Autodesk Inventor part; units mm, degrees
ref_plane "YZ Plane" through (0, 0, 0) normal (1, 0, 0) x (0, 1, 0)
ref_plane "XZ Plane" through (0, 0, 0) normal (0, 1, 0) x (-1, 0, 0)
ref_plane "XY Plane" through (0, 0, 0) normal (0, 0, 1) x (1, 0, 0)
sketch "Sketch1" plane through (0, 0, 0) normal (0, 0, 1) x (1, 0, 0)
  line L0 (-55.88, 39.751) -> (-55.88, -39.751)
  line L1 (-55.88, 39.751) -> (23.622, 39.751) construction
  line L2 (-55.88, -39.751) -> (55.88, -39.751)
  line L3 (55.88, -39.751) -> (55.88, 39.751)
  line L4 (55.88, 39.751) -> (-55.88, 39.751)
  line L5 (0, -55.6514) -> (0, 55.6514)
  line L6 (-78.232, 0) -> (78.232, 0)
  line L7 (-14.351, 39.751) -> (-14.351, 11.049)
  line L8 (-14.351, 11.049) -> (14.351, 11.049)
  line L9 (14.351, 11.049) -> (14.351, 39.751)
  point P0 (0, 0)
  dimension "d0" = 79.502
  dimension "d1" = 90
  dimension "d2" = 111.76
  dimension "d3" = 28.702
  dimension "d4" = 28.702
extrude "Extrusion1" add sketch "Sketch1" along normal blind 1.5875 contours L4 L7 L8 L5 L6 L0 | L6 L5 L2 L0 | L6 L3 L2 L5 | L5 L8 L9 L4 L3 L6
sketch "Sketch2" plane through (-41.656, -2.7227, 1.5875) normal (0, 0, 1) x (1, 0, 0)
  line L0 (97.536, -37.0283) -> (97.536, 37.0283)
  line L1 (-14.224, -37.0283) -> (97.536, -37.0283)
  line L2 (97.536, -37.0283) -> (97.536, 42.4737)
  line L3 (-14.224, -37.0283) -> (97.536, -37.0283)
  point P0 (0, 0)
  point P1 (83.312, 26.9797)
  point P2 (83.312, -21.2803)
  point P3 (97.536, 0)
  point P4 (41.656, -37.0283)
  dimension "d10" = 48.26
  dimension "d11" = 14.224
  dimension "d9" = 14.224
  dimension "d8" = 15.748
hole "Hole1" at (41.656, 24.257, 1.5875) at (41.656, -24.003, 1.5875) direction (0, 0, -1) diameter 5.5118 end through all
mirror "Mirror1" about plane through (0, 0, 0) normal (1, 0, 0) of "Hole1"
properties part number "DIFF_HOUSING_NO"
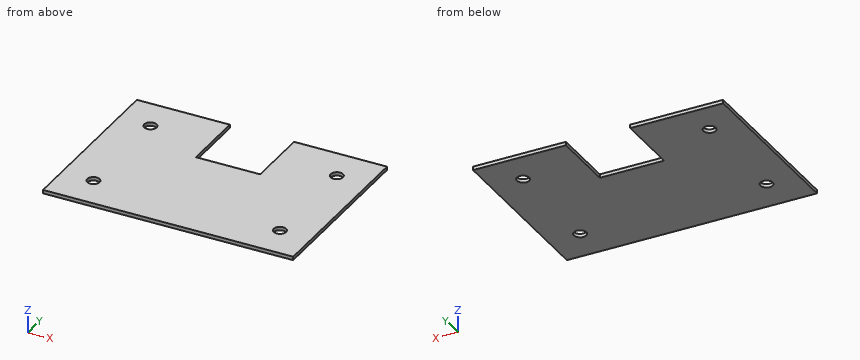
Read the model definition and answer for the solid it produces. Units are mm, in the model's axes. Give positions to 0.01 mm unless a question says otherwise; leave off trailing zeros. Order: outer loops, then holes, each group sorted by start corner. A loop starts at its lowest first (then second) coordinate and runs counter-clockwise, first axis right, second up.
(1) Find section B-B (z = 0.55). Give the vertices of the cut face in (x, y), plus the area to 3 significant figures.
(2) Find section A-A (y = 18). Give the vertices of the cut face in (x, z), plus the area to 3 significant figures.
(3) Straight lines are drawn through the part: L1, parallel to X at y = 31.5, z = 1.4; L2, parallel to Y at x = -43.5, z = 0.25; L3, parallel to Y at x = 4, z = 0.1. For each, find the intervals that lie inside material, in ascending order.
(4) Find section D-D (x = -7.5). Give the vertices of the cut face in (y, z).
(5) Given pin 1 (0.8 mm diameter, centred on x = 6, z = 0.5, fed in from +Y), flat-ended and moving along its own axis, determine where the tip first touches the part or whether it passes through.
(6) Find section C-C (y = -22.5). Give the vertices of the cut face in (x, z), plus the area to 3 significant figures.
Result sheet:
1. outline: (-55.88, -39.75) - (55.88, -39.75) - (55.88, 39.75) - (14.35, 39.75) - (14.35, 11.05) - (-14.35, 11.05) - (-14.35, 39.75) - (-55.88, 39.75) - close; hole circle Ø5.51 at (-41.66, -24); hole circle Ø5.51 at (-41.66, 24.26); hole circle Ø5.51 at (41.66, -24); hole circle Ø5.51 at (41.66, 24.26)
1. area: 7,970 mm2
2. outline: (-55.88, 0) - (-14.35, 0) - (-14.35, 1.59) - (-55.88, 1.59) - close; (14.35, 0) - (55.88, 0) - (55.88, 1.59) - (14.35, 1.59) - close
2. area: 132 mm2
3. L1: x = -55.88 to -14.35, 14.35 to 55.88
3. L2: y = -39.75 to -26.05, -21.95 to 22.21, 26.31 to 39.75
3. L3: y = -39.75 to 11.05
4. outline: (-39.75, 0) - (11.05, 0) - (11.05, 1.59) - (-39.75, 1.59) - close
5. pin 1: stops at y = 11.05
6. outline: (-55.88, 0) - (-43.97, 0) - (-43.97, 1.59) - (-55.88, 1.59) - close; (-39.35, 0) - (39.35, 0) - (39.35, 1.59) - (-39.35, 1.59) - close; (43.97, 0) - (55.88, 0) - (55.88, 1.59) - (43.97, 1.59) - close
6. area: 163 mm2
